from build123d import *

# Parameters (mm, degrees)
F0_R      = 14
F1_DEPTH  = 20
F2_SIZE   = 10
F4_DEPTH  = 38.6586394161
F5_R      = 13.8386431078
F6_F1_R   = 12
F6_F2_R   = 12
F7_W      = 49.8866699636
F7_H      = 41.0156846046
F8_DEPTH  = 38.5990254581
F10_DEPTH = 25


with BuildPart() as f1:
    # F0 (on Right) → F1 (new body)
    with BuildSketch(Plane.YZ):
        with BuildLine():
            Line((-15, 21.0786387324), (-15, 0))
            ThreePointArc((-15, 0), (0, -15), (15, 0))
            Line((15, 0), (15, 21.0786387324))
            Line((15, 21.0786387324), (-15, 21.0786387324))
        make_face()
        Circle(F0_R, mode=Mode.SUBTRACT)
    extrude(amount=F1_DEPTH)

    # F2
    f2_edges = [f1.edges().sort_by_distance(p)[0] for p in [
        (10, -15, 21.078639),
        (10, 15, 21.078639),
    ]]
    chamfer(f2_edges, length=F2_SIZE)

    # F3 (on face) → F4 (cut)
    with BuildSketch(Plane(origin=(0, 15, 0), x_dir=(-1, 0, 0), z_dir=(0, 1, 0))):
        with BuildLine():
            Line((-5.1145853621, 0), (0, 0))
            Line((0, 0), (0, 11.0786387324))
            ThreePointArc((0, 11.0786387324), (-2.8965213104, 5.6959282984), (-5.1145853621, 0))
        make_face()
        with BuildLine():
            Line((-20, 0), (-14.8854146379, 0))
            ThreePointArc((-14.8854146379, 0), (-17.1034786896, 5.6959282984), (-20, 11.0786387324))
            Line((-20, 11.0786387324), (-20, 0))
        make_face()
        with BuildLine():
            Line((-20, -15), (-12.5, -15))
            ThreePointArc((-12.5, -15), (-13.1198156851, -7.4088943941), (-14.8854146379, 0))
            Line((-14.8854146379, 0), (-20, 0))
            Line((-20, 0), (-20, -15))
        make_face()
        with BuildLine():
            Line((-7.5, -15), (0, -15))
            Line((0, -15), (0, 0))
            Line((0, 0), (-5.1145853621, 0))
            ThreePointArc((-5.1145853621, 0), (-6.8801843149, -7.4088943941), (-7.5, -15))
        make_face()
    extrude(amount=-F4_DEPTH, mode=Mode.SUBTRACT)

    # F5
    f5_edges = [f1.edges().sort_by_distance(p)[0] for p in [
        (10, 15, 11.078639),
        (10, -15, 11.078639),
    ]]
    fillet(f5_edges, radius=F5_R)

    # F6: fillet of radius 12 on 4 edges, made by hand

    # F6_f1
    f6_f1_edges = [f1.edges().sort_by_distance(p)[0] for p in [
        (0, -11.1582173276, 11.0786387324),
    ]]
    fillet(f6_f1_edges, radius=F6_F1_R)

    # F6_f2
    f6_f2_edges = [f1.edges().sort_by_distance(p)[0] for p in [
        (20, -11.1582173276, 11.0786387324),
    ]]
    fillet(f6_f2_edges, radius=F6_F2_R)

    # F7 (on Right) → F8 (cut, symmetric)
    with BuildSketch(Plane.YZ):
        with Locations((-1.9184369594, 39.5302809775)):
            Rectangle(F7_W, F7_H)
    extrude(amount=F8_DEPTH, both=True, mode=Mode.SUBTRACT)

    # F9 (on Right) → F10 (cut)
    with BuildSketch(Plane.YZ):
        with BuildLine():
            ThreePointArc((13.1383126183, 12.5615130593), (13.6820509432, 10.9110715325), (15.1701192952, 10.0137080727))
            ThreePointArc((15.1701192952, 10.0137080727), (15.5705478949, 10.9205773773), (16.2919620049, 11.6005161105))
            ThreePointArc((16.2919620049, 11.6005161105), (15.6366296494, 12.4697960372), (14.9349695532, 13.3021308235))
            ThreePointArc((14.9349695532, 13.3021308235), (14.111548562, 12.7501046734), (13.1383126183, 12.5615130593))
        make_face()
        with BuildLine():
            ThreePointArc((10.6842297635, 14.7055806807), (11.5139277039, 13.1787506551), (13.1383126183, 12.5615130593))
            ThreePointArc((13.1383126183, 12.5615130593), (13.3703783986, 13.5253078885), (13.9587913382, 14.3231331899))
            ThreePointArc((13.9587913382, 14.3231331899), (13.1587745188, 15.0614293201), (12.3197712741, 15.755101896))
            ThreePointArc((12.3197712741, 15.755101896), (11.6081510723, 15.0649195379), (10.6842297635, 14.7055806807))
        make_face()
        with BuildLine():
            ThreePointArc((11.1769736326, 16.5853929835), (10.7404739393, 15.6953238755), (10.6842297635, 14.7055806807))
            ThreePointArc((10.6842297635, 14.7055806807), (11.6081510723, 15.0649195379), (12.3197712741, 15.755101896))
            ThreePointArc((12.3197712741, 15.755101896), (11.7557050458, 16.1803398875), (11.1769736326, 16.5853929835))
        make_face()
        with BuildLine():
            ThreePointArc((7.8867469732, 16.3769988391), (8.9757373546, 15.022853888), (10.6842297635, 14.7055806807))
            ThreePointArc((10.6842297635, 14.7055806807), (10.7404739393, 15.6953238755), (11.1769736326, 16.5853929835))
            ThreePointArc((11.1769736326, 16.5853929835), (10.2579855481, 17.168975872), (9.3086054096, 17.7016910302))
            ThreePointArc((9.3086054096, 17.7016910302), (8.7316580559, 16.895535493), (7.8867469732, 16.3769988391))
        make_face()
        with BuildLine():
            ThreePointArc((8.0359187979, 18.3145846001), (7.7653618104, 17.3608792391), (7.8867469732, 16.3769988391))
            ThreePointArc((7.8867469732, 16.3769988391), (8.7316580559, 16.895535493), (9.3086054096, 17.7016910302))
            ThreePointArc((9.3086054096, 17.7016910302), (8.6776747824, 18.019377358), (8.0359187979, 18.3145846001))
        make_face()
        with BuildLine():
            ThreePointArc((-9.3086054096, 17.7016910302), (-8.7316580559, 16.895535493), (-7.8867469732, 16.3769988391))
            ThreePointArc((-7.8867469732, 16.3769988391), (-7.7903858604, 16.7677879095), (-7.7579855481, 17.168975872))
            ThreePointArc((-7.7579855481, 17.168975872), (-7.8284622538, 17.758396403), (-8.0359187979, 18.3145846001))
            ThreePointArc((-8.0359187979, 18.3145846001), (-8.6776747824, 18.019377358), (-9.3086054096, 17.7016910302))
        make_face()
        with BuildLine():
            ThreePointArc((-10.6842297635, 14.7055806807), (-8.9757373546, 15.022853888), (-7.8867469732, 16.3769988391))
            ThreePointArc((-7.8867469732, 16.3769988391), (-8.7316580559, 16.895535493), (-9.3086054096, 17.7016910302))
            ThreePointArc((-9.3086054096, 17.7016910302), (-10.2579855481, 17.168975872), (-11.1769736326, 16.5853929835))
            ThreePointArc((-11.1769736326, 16.5853929835), (-10.79186702, 15.8662578063), (-10.6587745188, 15.0614293201))
            ThreePointArc((-10.6587745188, 15.0614293201), (-10.6651464503, 14.883050353), (-10.6842297635, 14.7055806807))
        make_face()
        with BuildLine():
            ThreePointArc((-12.3197712741, 15.755101896), (-11.6081510723, 15.0649195379), (-10.6842297635, 14.7055806807))
            ThreePointArc((-10.6842297635, 14.7055806807), (-10.6651464503, 14.883050353), (-10.6587745188, 15.0614293201))
            ThreePointArc((-10.6587745188, 15.0614293201), (-10.79186702, 15.8662578063), (-11.1769736326, 16.5853929835))
            ThreePointArc((-11.1769736326, 16.5853929835), (-11.7557050458, 16.1803398875), (-12.3197712741, 15.755101896))
        make_face()
        with BuildLine():
            ThreePointArc((-13.1383126183, 12.5615130593), (-11.5139277039, 13.1787506551), (-10.6842297635, 14.7055806807))
            ThreePointArc((-10.6842297635, 14.7055806807), (-11.6081510723, 15.0649195379), (-12.3197712741, 15.755101896))
            ThreePointArc((-12.3197712741, 15.755101896), (-13.1587745188, 15.0614293201), (-13.9587913382, 14.3231331899))
            ThreePointArc((-13.9587913382, 14.3231331899), (-13.3703783986, 13.5253078885), (-13.1383126183, 12.5615130593))
        make_face()
        with BuildLine():
            ThreePointArc((-13.1366296494, 12.4697960372), (-13.137050427, 12.5156622681), (-13.1383126183, 12.5615130593))
            ThreePointArc((-13.1383126183, 12.5615130593), (-14.111548562, 12.7501046734), (-14.9349695532, 13.3021308235))
            ThreePointArc((-14.9349695532, 13.3021308235), (-15.6366296494, 12.4697960372), (-16.2919620049, 11.6005161105))
            ThreePointArc((-16.2919620049, 11.6005161105), (-15.5705478949, 10.9205773773), (-15.1701192952, 10.0137080727))
            ThreePointArc((-15.1701192952, 10.0137080727), (-13.7109770476, 10.8754742198), (-13.1366296494, 12.4697960372))
        make_face()
    extrude(amount=F10_DEPTH, mode=Mode.SUBTRACT)


solid = f1.part
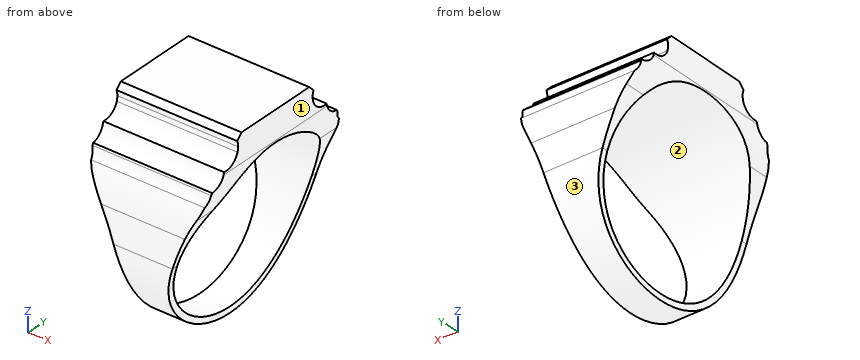
Read the model definition and answer for the solid it produces. Units are mm, in the model's axes. Face numbers are marked on the shaded views. Coordinates: 2 decimals unless noted, no trailing zeros. Loops run counter-clockwise (first coordinate to the right, second up) from the corner with the lowest first, then second, coordinate; pieces in that order, holes last. Notation, with made-up numbers: (-21.5, -33) -> (-16.5, -33) arc R22 ccw to (-16.5, -24) -> close; hole circle Ø10 at (-2.75, 20.5). An arc over 180 degrees is marked (long way). Write item = value, one per line. Start each with the question number.
1) The part is cut by section D-D, the plane z = -2. Determine the outline of the cut face in (x, y), plus the area to 3 significant figures.
2) The part is cut by section C-C, the plane x = 4.25. Determine the outline of the cut face in (y, z).
3) Given P1, Ø5, axis at y = 7, z = -10, coming from the +X side; P2, Ø5, axis at x = 10.5, z = -5, coming from the +Y side; P3, Ø4, axis at x = 13, z = 10, coming from the +Y side, each flat-ended and moving along its own axis, determine where each tip first touches the part or whether it passes through.
4) The part is cut by section A-A, the plane y = 2. Determine the outline of the cut face in (x, z), plus the area to 3 significant figures.
5) Find the intervals of material crossed by L1, parallel to Z at x = 8.5, y = 0; L2, parallel to Y at x = 8.25, z = 1; L3, parallel to Z at x = 12, y = 12.5, in increasing order. Write a range as from..to.
6) The mould has two halves that part along Z. Classify the marked faces 1, 2 and 3: pulls with the +Z half, pulls with the -Z half, needs draft (parallel to the pull), parting line crosses it, or undercut.
7) The part is cut by section B-B, the plane z = -12. Determine the outline of the cut face in (x, y).
Result:
q1.outline = (5.71, -14.87) -> (14.29, -14.87) -> (14.29, -13.86) -> (5.71, -13.86) -> close; (5.71, 13.86) -> (14.29, 13.86) -> (14.29, 14.87) -> (5.71, 14.87) -> close
q1.area = 17.3 mm²
q2.outline = (-15, 2.47) -> (-13.78, 2.47) arc R14 cw to (13.78, 2.47) -> (15, 2.47) -> (15, 5.35) arc R13.84 ccw to (13.96, 10.62) arc R2.5 cw to (13.14, 12.27) arc R13.84 ccw to (12.97, 12.57) arc R2.5 cw to (10.68, 14.71) arc R2.5 cw to (7.95, 18.13) -> (7.06, 19.02) -> (-7.06, 19.02) -> (-7.95, 18.13) arc R2.5 cw to (-10.68, 14.71) arc R2.5 cw to (-12.97, 12.57) arc R13.84 ccw to (-13.14, 12.27) arc R2.5 cw to (-13.96, 10.62) arc R13.84 ccw to (-15, 5.35) -> close
q3.P1 = 12.75
q3.P2 = 14.79
q3.P3 = 14.74
q4.outline = (0, 14.3) arc R12 ccw to (0.01, 13.86) -> (19.99, 13.86) arc R12 ccw to (20, 14.3) -> (20, 19.02) -> (0, 19.02) -> close; (7.48, -13.86) arc R50 cw to (7.5, -14.87) -> (12.5, -14.87) arc R50 cw to (12.52, -13.86) -> close
q4.area = 108 mm²
q5.L1 = -15..-14, 14..19.02
q5.L2 = -15..-13.96, 13.96..15
q5.L3 = -8.29..-6.3, 6.3..12.65
q6.face_1 = needs draft
q6.face_2 = undercut
q6.face_3 = pulls with the -Z half
q7.outline = (7.39, -9) -> (12.61, -9) -> (12.61, -7.21) -> (7.39, -7.21) -> close; (7.39, 7.21) -> (12.61, 7.21) -> (12.61, 9) -> (7.39, 9) -> close
